Autodesk Inventor part; units mm, degrees
ref_plane "YZ Plane" through (0, 0, 0) normal (1, 0, 0) x (0, 1, 0)
ref_plane "XZ Plane" through (0, 0, 0) normal (0, 1, 0) x (-1, 0, 0)
ref_plane "XY Plane" through (0, 0, 0) normal (0, 0, 1) x (1, 0, 0)
sketch "Sketch1" plane through (0, 0, 0) normal (0, 1, 0) x (-1, 0, 0)
  circle A0 centre (0, 0) radius 2.45
  dimension "d0" = 4.9
extrude "Extrusion1" add sketch "Sketch1" along normal blind 20
sketch "Sketch2" plane through (0, 20, 0) normal (0, 1, 0) x (1, 0, 0)
  circle A0 centre (0, 0) radius 3.5
  dimension "d3" = 7
extrude "Extrusion2" add sketch "Sketch2" along normal blind 2
thread "Thread1"
sketch "Sketch3" plane through (0, 22, 0) normal (0, 1, 0) x (1, 0, 0)
  line L0 (0.866, 1.5) -> (1.7321, 0)
  line L1 (1.7321, 0) -> (0.866, -1.5)
  line L2 (0.866, -1.5) -> (-0.866, -1.5)
  line L3 (-0.866, -1.5) -> (-1.7321, 0)
  line L4 (-1.7321, 0) -> (-0.866, 1.5)
  line L5 (-0.866, 1.5) -> (0.866, 1.5)
  point P0 (0, 0)
  point P1 (0, 0)
  dimension "d8" = 3
extrude "Extrusion3" cut sketch "Sketch3" against normal blind 1
equation "\"BendRadius\" = Thickness"
equation "\"BendReliefWidth\" = Thickness"
equation "\"BendReliefDepth\" = 0.5 * Thickness"
equation "\"CornerReliefSize\" = 4 * Thickness"
equation "\"MinimumRemnant\" = 2 * Thickness"
equation "\"TransitionRadius\" = BendRadius"
equation "\"JacobiRadiusSize\" = BendRadius"
equation "\"GapSize\" = Thickness"
properties part number "perno_simple"
Geometry: final body of the model. Coordinates: model frame, mm. A direction names the side the tool comes from. Round coordinates to 2 decimals unless told otherwise and drop trailing zeros. Loops run counter-clockwise (first coordinate to the right, second up) from the corner with the lowest first, then second, coordinate; pieces in that order, holes last. Notation, with made-up numbers: (32, 81.5) - (40, 81.5) arc R22 cw to (40, 115.5) - close; hole circle Ø10 at (38, -29). An arc over 180 degrees is marked (long way). Write each question's results on one line, items separated by ' | '. Start each with the question number.
1) Line query: probe 1 along Y at (x, z) = (-1, -0.5); probe 2 along Y at (x, z) = (3.25, -0.5); probe 3 along Z at (x, y) = (-2.5, 20.25). Output: solid intervals per line, ascending. Write a range as [from, to].
2) Access query for faces 1 (the face through (0, 22, 2)), 2 (the face through (0, 21, 0)), 3 (the face through (2, 20, 2)). Directions: +Z, -Z, +X, -X, +Y, -Y. A direction counts if a zero-diameter tool reaches every point of the face in a straight line with its end or side. Return the directions, or none.
3) Cut plane B-B on z = 2. Return loops of the section in (x, y).
4) Cut plane A-A on x = 0. Return loops of the section in (y, z), then the cut area to 3 significant figures.
5) Cut plane C-C on y = 4. Return loops of the section in (x, z), then the cut area to 3 significant figures.
6) Cut plane D-D on x = -1.25. Return loops of the section in (y, z), then the cut area to 3 significant figures.
7) First-contact query: P1, Ø1.5, axis at x = 2, y = 3.5, coming from the -Z side; P2, Ø1, axis at y = 16, z = 2.5, coming from the -X side; P3, Ø0.5, axis at x = -0.5, y = 21.5, coming from the +Z side. Flat tips, straight axial feed; report the tip coordinate or a pass-through.
Verdict:
1) probe 1: y = [0, 21] | probe 2: y = [20, 22] | probe 3: z = [-2.45, 2.45]
2) face 1: +Z, -Z, +X, -X, +Y | face 2: +Y | face 3: -Y
3) outline: (-2.87, 20) - (-1.42, 20) - (-1.42, 0) - (1.42, 0) - (1.42, 20) - (2.87, 20) - (2.87, 22) - (-2.87, 22) - close
4) outline: (0, -2.45) - (20, -2.45) - (20, -3.5) - (22, -3.5) - (22, -1.5) - (21, -1.5) - (21, 1.5) - (22, 1.5) - (22, 3.5) - (20, 3.5) - (20, 2.45) - (0, 2.45) - close | area: 109 mm2
5) outline: circle Ø4.9 at (0, 0) | area: 18.9 mm2
6) outline: (0, -2.11) - (20, -2.11) - (20, -3.27) - (22, -3.27) - (22, -0.83) - (21, -0.83) - (21, 0.83) - (22, 0.83) - (22, 3.27) - (20, 3.27) - (20, 2.11) - (0, 2.11) - close | area: 95.7 mm2
7) P1: stops at z = -2.11 | P2: stops at x = -1.42 | P3: stops at z = 3.49
